Check sheet for the modelled part. Datum: model origin and axes. Units: mm. Round coordinates to 2 decimals unless told otherwise and drop trailing zeros. Loops run counter-clockwise (first coordinate to the right, second up) from the corner with the lowest first, then second, coordinate; pieces in that order, holes last. Notation, with made-up numbers: (36.5, 33.25) -> (87.5, 33.25) arc R14 cw to (87.5, 41.25) -> close; hole circle Ø2 at (52, 62.5). An arc over 180 degrees is marked (long way). Return JSON: item names as keys, results as strings.
from build123d import *

# Parameters (mm, degrees)
SKETCH1_W           = 40
SKETCH1_H           = 5
BOSS_EXTRUDE2_DEPTH = 5
SKETCH2_W           = 25.4
SKETCH2_H           = 5.4
CUT_EXTRUDE1_DEPTH  = 5


with BuildPart() as part:
    # Sketch1 → Boss-Extrude2 (new body)
    with BuildSketch(Plane.XY):
        Polygon((-159, 330), (-188, 330), (-188, 0), (-159, 0), (-119, 0), (-96.1, 0), (-96.1, 6.8), (-97.5, 6.8), (-97.5, 10), (-96.1, 10), (-96.1, 17), (-91.9, 17), (-91.9, 10), (-90.5, 10), (-90.5, 6.8), (-91.9, 6.8), (-91.9, 0), (-69, 0), (-29, 0), (0, 0), (0, 330), (-29, 330), (-69, 330), (-91.9, 330), (-91.9, 323.2), (-90.5, 323.2), (-90.5, 320), (-91.9, 320), (-91.9, 313), (-96.1, 313), (-96.1, 320), (-97.5, 320), (-97.5, 323.2), (-96.1, 323.2), (-96.1, 330), (-119, 330), align=None)
        with Locations((-49, 332.5)):
            Rectangle(SKETCH1_W, SKETCH1_H)
        with Locations((-139, 332.5)):
            Rectangle(SKETCH1_W, SKETCH1_H)
        with Locations((-49, -2.5)):
            Rectangle(SKETCH1_W, SKETCH1_H)
        with Locations((-139, -2.5)):
            Rectangle(SKETCH1_W, SKETCH1_H)
    extrude(amount=BOSS_EXTRUDE2_DEPTH)

    # Sketch2 → Cut-Extrude1 (cut)
    with BuildSketch(Plane(origin=(0, 0, 0), x_dir=(-1, 0, 0), z_dir=(0, 0, -1))):
        with Locations((30.5, 197.500001815)):
            Rectangle(SKETCH2_W, SKETCH2_H)
        with Locations((157.5, 174.000000001)):
            Rectangle(SKETCH2_W, SKETCH2_H)
        with Locations((30.4, 150.500001815)):
            Rectangle(SKETCH2_W, SKETCH2_H)
        with Locations((157.5, 127)):
            Rectangle(SKETCH2_W, SKETCH2_H)
        with Locations((30.5, 103.500001815)):
            Rectangle(SKETCH2_W, SKETCH2_H)
        with Locations((157.5, 80)):
            Rectangle(SKETCH2_W, SKETCH2_H)
    extrude(amount=-CUT_EXTRUDE1_DEPTH, mode=Mode.SUBTRACT)


solid = part.part
Q1. Material ranges on line 1 (Y direction, x = -21.5, z = 0.85); line 2 (Y direction, x = -160, z = 4.05); line 3 (X direction, y = 152.5, z = 4.5), recorded low to high.
Results list:
{"line 1": "0 to 100.8, 106.2 to 147.8, 153.2 to 194.8, 200.2 to 330", "line 2": "0 to 77.3, 82.7 to 124.3, 129.7 to 171.3, 176.7 to 330", "line 3": "-188 to -43.1, -17.7 to 0"}
Q2. Section check B-B (x = -75). Record the boundary of the cut face in (y, z), then the cut area to 3 significant figures.
Results list:
{"outline": "(0, 0) -> (330, 0) -> (330, 5) -> (0, 5) -> close", "area": "1,650 mm^2"}
Q3. Go/stop test with flat-tipped pins: pin 1 (8 mm diameter, centred on x = -148, y = 164, fed in from -Z); pin 2 (1.1 mm diameter, centred on x = -96.5, z = 3.5, fed in from +Y); pin 3 (2.5 mm diameter, centred on x = -162, z = 2, fed in from -Y). Record where each tip stops, or that it passes through.
Results list:
{"pin 1": "z = 0", "pin 2": "y = 330", "pin 3": "y = 0"}
Q4. Section check A-A (z = 3.65). Count the separate pieces of the cut face and the enclosed holes in it, then the cut area to 3 significant figures.
Results list:
{"separate pieces": "1", "enclosed holes": "6", "area": "61,900 mm^2"}
